from build123d import *

# Parameters (mm, degrees)
SKETCH1_W           = 17.145
SKETCH1_H           = 17.145
BOSS_EXTRUDE1_DEPTH = 5.08
SKETCH2_R           = 1.27
CUT_EXTRUDE1_DEPTH  = 6.08
SKETCH3_R           = 2.54
CUT_EXTRUDE4_DEPTH  = 2.54
SKETCH4_W           = 6.307704678
SKETCH4_H           = 17.145
BOSS_EXTRUDE2_DEPTH = 17.78
SKETCH5_W           = 2.54
SKETCH5_H           = 17.145
BOSS_EXTRUDE3_DEPTH = 5.08
CHAMFER1_SIZE       = 3.175
BOSS_EXTRUDE4_DEPTH = 2.54
BOSS_EXTRUDE5_DEPTH = 2.54


with BuildPart() as part:
    # Sketch1 → Boss-Extrude1 (new body)
    with BuildSketch(Plane.XY):
        with Locations((8.5725, -8.5725)):
            Rectangle(SKETCH1_W, SKETCH1_H)
    extrude(amount=BOSS_EXTRUDE1_DEPTH)

    # Sketch2 → Cut-Extrude1 (cut, through all)
    with BuildSketch(Plane(origin=(0, 0, 0), x_dir=(-1, 0, 0), z_dir=(0, 0, -1))):
        with Locations((-8.89, -2.5908)):
            Circle(SKETCH2_R)
        with Locations((-8.89, -14.5288)):
            Circle(SKETCH2_R)
    extrude(amount=-CUT_EXTRUDE1_DEPTH, mode=Mode.SUBTRACT)

    # Sketch3 → Cut-Extrude4 (cut)
    with BuildSketch(Plane(origin=(0, 0, 0), x_dir=(-1, 0, 0), z_dir=(0, 0, -1))):
        with Locations((-8.89, -2.5908)):
            Circle(SKETCH3_R)
        with Locations((-8.89, -14.5288)):
            Circle(SKETCH3_R)
    extrude(amount=-CUT_EXTRUDE4_DEPTH, mode=Mode.SUBTRACT)

    # Sketch4 → Boss-Extrude2 (add)
    with BuildSketch(Plane(origin=(0, 0, 0), x_dir=(-1, 0, 0), z_dir=(0, 0, -1))):
        with Locations((-3.153852339, -8.5725)):
            Rectangle(SKETCH4_W, SKETCH4_H)
    extrude(amount=BOSS_EXTRUDE2_DEPTH)

    # Sketch5 → Boss-Extrude3 (add)
    with BuildSketch(Plane.ZY):
        with Locations((3.81, -8.5725)):
            Rectangle(SKETCH5_W, SKETCH5_H)
    extrude(amount=BOSS_EXTRUDE3_DEPTH)

    # Chamfer1
    chamfer1_edges = [part.edges().sort_by_distance(p)[0] for p in [
        (0, -8.5725, -17.78),
    ]]
    chamfer(chamfer1_edges, length=CHAMFER1_SIZE)

    # Sketch7 → Boss-Extrude4 (add)
    with BuildSketch(Plane(origin=(0, 0, 0), x_dir=(1, 0, 0), z_dir=(0, 1, 0))):
        Polygon((-5.08, -2.54), (0, 14.605), (0, -2.54), align=None)
    extrude(amount=-BOSS_EXTRUDE4_DEPTH)

    # Sketch8 → Boss-Extrude5 (add)
    with BuildSketch(Plane.XZ.offset(17.145)):
        Polygon((0, 2.54), (-5.08, 2.54), (0, -14.605), align=None)
    extrude(amount=-BOSS_EXTRUDE5_DEPTH)


solid = part.part
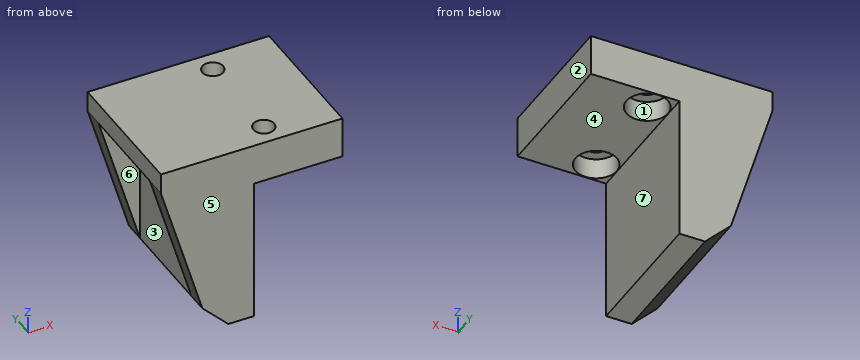
Could you check a few things on this model? Use its own coordinates, in mm. Face numbers are marked on the shaded views. A direction names the side the tool comes from. Give positions to 0.01 mm unless a question says otherwise; leave off trailing zeros. Order: outer loops, then holes, each group sorted by start corner. A loop starts at its lowest first (then second) coordinate and runs counter-clockwise, first axis right, second up.
1. Suppose I cut it at C-C (z = -6). Write out the boundary of the cut face in (x, y) (3 decimals).
Answers below:
outline: (-2.55, -17.145) - (6.308, -17.145) - (6.308, 0) - (-2.55, 0) - (-2.55, -2.54) - (0, -2.54) - (0, -14.605) - (-2.55, -14.605) - close
2. Suppose I cut it at A-A (x = 8.89). Write out the boundary of the cut face in (y, z) (3 decimals), plus the area to 3 significant figures.
Answers below:
outline: (-17.145, 0) - (-17.069, 0) - (-17.069, 2.54) - (-15.799, 2.54) - (-15.799, 5.08) - (-17.145, 5.08) - close; (-13.259, 2.54) - (-11.989, 2.54) - (-11.989, 0) - (-5.131, 0) - (-5.131, 2.54) - (-3.861, 2.54) - (-3.861, 5.08) - (-13.259, 5.08) - close; (-1.321, 2.54) - (-0.051, 2.54) - (-0.051, 0) - (0, 0) - (0, 5.08) - (-1.321, 5.08) - close
area: 48.4 mm2
3. For pin 1 (2 mm diameter, centred on y = -8.5, z = -15, fed in from +X); pin 2 (2 mm diameter, centred on x = 10, y = -4.5, fed in from -Z); pin 3 (2.5 mm diameter, centred on x = -3, y = -6, fed in from -Z); pin 4 (2 mm diameter, centred on x = 8.89, y = -2.59, fed in from +Z), each with a flat end and sliding along its axis, tell me the tip position at first contact or that it passes through.
Answers below:
pin 1: stops at x = 6.31
pin 2: stops at z = 0
pin 3: stops at z = 2.54
pin 4: passes through
4. Suppose I cut it at B-B (y = -6.25). Write out the boundary of the cut face in (x, z) (3 decimals).
Answers below:
outline: (-5.08, 2.54) - (0, 2.54) - (0, -14.605) - (3.175, -17.78) - (6.308, -17.78) - (6.308, 0) - (17.145, 0) - (17.145, 5.08) - (-5.08, 5.08) - close
5. Suppose I cut it at D-D (z = 1.25). Write out the boundary of the cut face in (x, y) (3 decimals).
Answers below:
outline: (-4.698, -17.145) - (17.145, -17.145) - (17.145, 0) - (-4.698, 0) - (-4.698, -2.54) - (0, -2.54) - (0, -14.605) - (-4.698, -14.605) - close; hole circle Ø5.08 at (8.89, -14.529); hole circle Ø5.08 at (8.89, -2.591)
6. I need wall thicknesses on L1, parallel to Y at x = 8.89, z = 3.25 (3 decimals); L2, parallel to Y at x = -2, z = 0.5 (3 decimals); L3, parallel to X at y = -13.5, z = -14.5. Which ranges of each line are inside material? Lowest first, please.
Answers below:
L1: y = -17.145 to -15.799, -13.259 to -3.861, -1.321 to 0
L2: y = -17.145 to -14.605, -2.54 to 0
L3: x = 0 to 6.31
7. Which directions (+Z, -Z, +X, -X, +Y, -Y) give clear straight access to the entire face, cutting with the end or side of a thin tool? Please do the marked faces 1, 2, 3 and 4.
Answers below:
face 1: -Z
face 2: +Z, -Z, +X, +Y, -Y
face 3: -Z, -X
face 4: -Z, +X, +Y, -Y
8. Thinking about a two-plate mould opening in Y: for the marked faces 5, 6 and 7, which applies, +Y half, -Y half, draft (parallel to the pull), parting line (faces both ways), or undercut?
Answers below:
face 5: -Y half
face 6: undercut
face 7: draft
